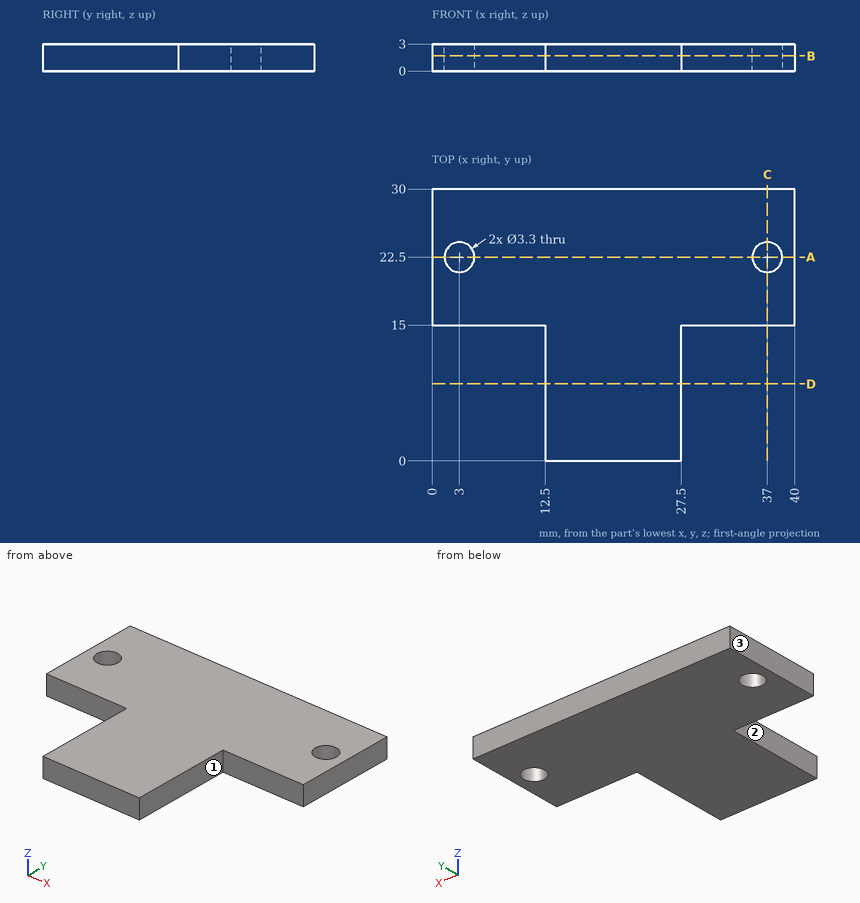
Answer from the drawing. Dimensions are ordinates in mm from the lowest x, y and z of the part. A direction names the side the tool comes from. Round coordinates to 2 decimals unless told otherwise and drop trailing zeros. Order: outer loops, then holes, each group sorted by start corner. A loop starts at its lowest first (then second) coordinate and runs counter-clockwise, first axis right, second up. Notation, with made-up numbers: (66.25, 28.25) -> (75.25, 28.25) arc R26 ccw to (75.25, 56.25) -> close; hole circle Ø4 at (25.5, 33). An arc over 180 degrees is marked (long way). Answer as CSV lines item,"result".
Q1. A cutting plane is placed at D-D on y = 8.5. Determine the outline of the cut face in (x, z), plus the area to 3 significant figures.
Computed values:
outline,"(12.5, 0) -> (27.5, 0) -> (27.5, 3) -> (12.5, 3) -> close"
area,"45.0 mm^2"
Q2. Which of the six approach directions +Z, -Z, +X, -X, +Y, -Y give full straight-line access (tool end or side, diameter ignored) to the marked faces 1, 2 and 3?
Computed values:
face 1,"+Z, -Z, +X, -Y"
face 2,"+Z, -Z, -X, -Y"
face 3,"+Z, -Z, -X, +Y, -Y"
Q3. Consider line 1 (Y direction, x = 37, z = 2.4); line 2 (X direction, y = 23.5, z = 1.6); line 3 (X direction, y = 22, z = 1.75). Determine where each line is inside the solid, lowest interval first. Write a range as from..to.
Computed values:
line 1,"y = 15..20.85, 24.15..30"
line 2,"x = 0..1.69, 4.31..35.69, 38.31..40"
line 3,"x = 0..1.43, 4.57..35.43, 38.57..40"
Q4. A cutting plane is placed at B-B on z = 1.7. Determine the outline of the cut face in (x, y).
Computed values:
outline,"(0, 15) -> (12.5, 15) -> (12.5, 0) -> (27.5, 0) -> (27.5, 15) -> (40, 15) -> (40, 30) -> (0, 30) -> close; hole circle Ø3.3 at (3, 22.5); hole circle Ø3.3 at (37, 22.5)"
Q5. Given pin 1 (0.9 mm diameter, centred on x = 34.5, z = 1, fed in from -Y), flat-ended and moving along its own axis, determine where the tip first touches the part or whether it passes through.
Computed values:
pin 1,"stops at y = 15"
Q6. A cutting plane is placed at C-C on x = 37. Determine the outline of the cut face in (y, z).
Computed values:
outline,"(15, 0) -> (20.85, 0) -> (20.85, 3) -> (15, 3) -> close; (24.15, 0) -> (30, 0) -> (30, 3) -> (24.15, 3) -> close"
Q7. A cutting plane is placed at A-A on y = 22.5. Determine the outline of the cut face in (x, z).
Computed values:
outline,"(0, 0) -> (1.35, 0) -> (1.35, 3) -> (0, 3) -> close; (4.65, 0) -> (35.35, 0) -> (35.35, 3) -> (4.65, 3) -> close; (38.65, 0) -> (40, 0) -> (40, 3) -> (38.65, 3) -> close"
